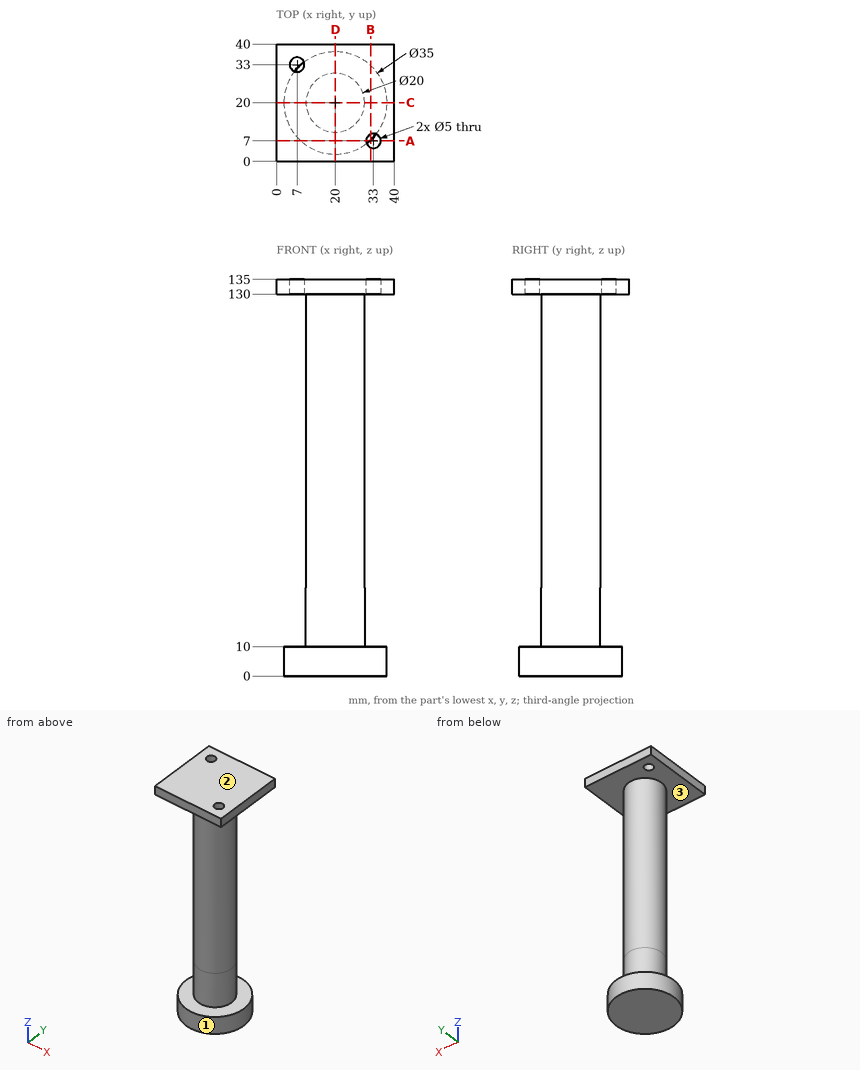
Geometry check sheet. Reference: drawing and pictorial views, mm from the part's lowest x, y, z. Round coordinates to 2 decimals unless told otherwise and drop trailing zeros. Loops run counter-clockwise (first coordinate to the right, second up) from the corner with the lowest first, then second, coordinate; pieces in that order, holes last. Notation, with made-up numbers: (-4, 36.25) - (36, 36.25) arc R27 cw to (36, 72.25) - close; hole circle Ø1 at (65, 61.25). An arc over 180 degrees is marked (long way). Use a Markdown table: item, result.
Q1. Material ranges on line 1 (Y direction, x = 7, z = 132); line 2 (Z direction, x = 33, y = 14.5); line 3 (Z direction, x = 32, y = 4.5), recorded low to high.
Solutions:
| item | result |
|---|---|
| line 1 | y = 0 to 30.5, 35.5 to 40 |
| line 2 | z = 0 to 10, 130 to 135 |
| line 3 | z = 130 to 135 |
Q2. Cross-section at B-B on x = 32. Record the cut outline in (y, z), plus the area to 3 significant figures.
Solutions:
| item | result |
|---|---|
| outline | (0, 130) - (4.71, 130) - (4.71, 135) - (0, 135) - close; (7.26, 0) - (32.74, 0) - (32.74, 10) - (7.26, 10) - close; (9.29, 130) - (40, 130) - (40, 135) - (9.29, 135) - close |
| area | 432 mm2 |
Q3. Go/stop test with flat-tipped pins: P1, Ø2, axis at x = 21.5, z = 21, coming from the -Y side; P2, Ø4, axis at x = 28.5, z = 48.5, coming from the +Y side; P3, Ø6, axis at x = 16.5, z = 80.5, coming from the +Y side. Record where each tip stops, or that it passes through.
Solutions:
| item | result |
|---|---|
| P1 | stops at y = 10.01 |
| P2 | stops at y = 27.6 |
| P3 | stops at y = 29.99 |
Q4. Draft check along Z on the marked faces 1, 2 and 3. Enter one of: released by +Z, released by -Z, zero draft, split by the parting line, or undercut.
Solutions:
| item | result |
|---|---|
| face 1 | zero draft |
| face 2 | released by +Z |
| face 3 | undercut |
Q5. Cross-section at A-A on y = 7. Record the cut outline in (x, z), plus the area to 3 significant figures.
Solutions:
| item | result |
|---|---|
| outline | (0, 130) - (30.5, 130) - (30.5, 135) - (0, 135) - close; (8.28, 0) - (31.72, 0) - (31.72, 10) - (8.28, 10) - close; (35.5, 130) - (40, 130) - (40, 135) - (35.5, 135) - close |
| area | 409 mm2 |
Q6. Cross-section at C-C on y = 20. Record the cut outline in (x, z), plus the area to 3 significant figures.
Solutions:
| item | result |
|---|---|
| outline | (0, 130) - (10, 130) - (10, 10) - (2.5, 10) - (2.5, 0) - (37.5, 0) - (37.5, 10) - (30, 10) - (30, 130) - (40, 130) - (40, 135) - (0, 135) - close |
| area | 2,950 mm2 |
